```python
from build123d import *

# Parameters (mm, degrees)
F0_R     = 12.5
F1_DEPTH = 50
F2_T     = -1
F3_R     = 0.1


with BuildPart() as f1:
    # F0 (on Top) → F1 (new body)
    with BuildSketch(Plane.XY):
        Circle(F0_R)
    extrude(amount=F1_DEPTH)

    # F2
    f2_openings = [f1.faces().sort_by_distance(p)[0] for p in [
        (0, 0, 50),
    ]]
    offset(amount=F2_T, openings=f2_openings)

    # F3
    f3_edges = [f1.edges().sort_by_distance(p)[0] for p in [
        (-12.5, 0, 0),
    ]]
    fillet(f3_edges, radius=F3_R)


solid = f1.part
```
Could you check a few things on this model? Use its own coordinates, in mm. A direction names the side the tool comes from. Round coordinates to 2 decimals unless told otherwise and drop trailing zeros. Loops run counter-clockwise (first coordinate to the right, second up) from the corner with the lowest first, then second, coordinate; pieces in that order, holes last. Notation, with made-up numbers: M 3.25,9 L 49.25,9 A21 cw 49.25,23 Z; hole C 20,89.25 d3. An arc over 180 degrees is marked long. Answer as CSV lines item,"result".
1) For pin 1 Ø8 at (y, z) = (-4.5, 29) entering from -X; pin 2 Ø2 at (x, y) = (-3, -3) entering from +Z; pin 3 Ø8 at (y, z) = (-8.5, 18) entering from -X, each with a flat end and sliding along its axis, tell me the tip position at first contact or that it passes through.
From the geometry:
pin 1,"x = -12.49"
pin 2,"z = 1"
pin 3,"x = -11.66"
2) Imagine slicing it at B-B on z = 33.5. List the corners of the cut face in (x, y) for me.
From the geometry:
outline,"C 0,0 d25; hole C 0,0 d23"
3) If I drill on probe 1 along Y at (x, z) = (0, 28); probe 2 along Y at (x, z) = (-4.5, 23); probe 3 along X at (y, z) = (-1.5, 15), over which ranges is the centre line in solid material (lowest first)?
From the geometry:
probe 1,"-12.5 to -11.5, 11.5 to 12.5"
probe 2,"-11.66 to -10.58, 10.58 to 11.66"
probe 3,"-12.41 to -11.4, 11.4 to 12.41"
4) Imagine slicing it at A-A on y = 0. List the corners of the cut face in (x, z) for me, and give its area (3 significant figures).
From the geometry:
outline,"M -12.5,0.1 A0.1 ccw -12.4,0 L 12.4,0 A0.1 ccw 12.5,0.1 L 12.5,50 L 11.5,50 L 11.5,1 L -11.5,1 L -11.5,50 L -12.5,50 Z"
area,"123 mm^2"
5) Which directions (+Z, -Z, +X, -X, +Y, -Y) give clear straight access to the entire face, cutting with the end or side of a thin tool? Please do faces 1 (the cylindrical face through (-1.5, 11.4, 25.2)), 2 (the flat face through (11, -4, 50)).
From the geometry:
face 1,"+Z"
face 2,"+Z, +X, -X, +Y, -Y"
